CAD build for the part. Positions are in the model's coordinates, mm. A direction names the side the tool comes from. Give positions to 0.01 mm unless a question says otherwise; leave off trailing zeros. Write each loop counter-clockwise with the first axis right and the second up, starting at its lowest first coordinate (ties: lowest second). Pieces come first, ordered by that corner, then holes. Notation, with made-up numbers: (-27.75, -33.75) -> (-8.75, -33.75) arc R13 ccw to (-8.75, -25.75) -> close; hole circle Ø8 at (-34.5, 12). An arc over 180 degrees is marked (long way). Answer as a JSON object with one key per item and string values.
```python
from build123d import *

# Parameters (mm, degrees)
BOSS_EXTRUDE1_DEPTH      = 50
BOSS_EXTRUDE1_DEPTH_BACK = 50
SKETCH2_R                = 100
CUT_EXTRUDE1_DEPTH       = 50
CUT_EXTRUDE1_DEPTH_BACK  = 50
SKETCH3_R                = 75
CUT_EXTRUDE2_DEPTH       = 40
CUT_EXTRUDE2_DEPTH_BACK  = 40
SKETCH4_R                = 200


with BuildPart() as part:
    # Sketch2 → Boss-Extrude1 (new, two sides: drawn at the far end of the back side and taken through both)
    with BuildSketch(Plane.XY.offset(-BOSS_EXTRUDE1_DEPTH_BACK)):
        Circle(SKETCH2_R)
        with BuildLine():
            Line((600, 100), (0, 100))
            ThreePointArc((0, 100), (70.710678119, 70.710678119), (100, 0))
            ThreePointArc((100, 0), (70.710678119, -70.710678119), (0, -100))
            Line((0, -100), (600, -100))
            ThreePointArc((600, -100), (500, 0), (600, 100))
        make_face()
        with Locations((600, 0)):
            Circle(SKETCH2_R)
    extrude(amount=BOSS_EXTRUDE1_DEPTH + BOSS_EXTRUDE1_DEPTH_BACK)

    # Sketch3 → Cut-Extrude1 (cut, two sides: drawn at the far end of the back side and taken through both)
    with BuildSketch(Plane.XY.offset(-CUT_EXTRUDE1_DEPTH_BACK)):
        Circle(SKETCH3_R)
    extrude(amount=CUT_EXTRUDE1_DEPTH + CUT_EXTRUDE1_DEPTH_BACK, mode=Mode.SUBTRACT)

    # Sketch4 → Cut-Extrude2 (cut, two sides: drawn at the far end of the back side and taken through both)
    with BuildSketch(Plane.XY.offset(-CUT_EXTRUDE2_DEPTH_BACK)):
        Circle(SKETCH4_R)
    extrude(amount=CUT_EXTRUDE2_DEPTH + CUT_EXTRUDE2_DEPTH_BACK, mode=Mode.SUBTRACT)


solid = part.part
```
1) Slice it at A-A (y = 0). List the corners of the cut face in (x, z), then the cut area to 3 significant figures.
Model answer:
{"outline": "(-100, -50) -> (-75, -50) -> (-75, -40) -> (-100, -40) -> close; (-100, 40) -> (-75, 40) -> (-75, 50) -> (-100, 50) -> close; (75, -50) -> (700, -50) -> (700, 50) -> (75, 50) -> (75, 40) -> (200, 40) -> (200, -40) -> (75, -40) -> close", "area": "53,000 mm2"}
2) Pin check, flat tips, straight feed: pin 1 (1.5 mm diameter, centred on y = 77.5, z = 8.5, fed in from -X); pin 2 (5 mm diameter, centred on y = 9.5, z = -22.5, fed in from +X); pin 3 (1.5 mm diameter, centred on y = 42.5, z = -19, fed in from +X). Stop position of each tip, or through.
Model answer:
{"pin 1": "stops at x = 184.06", "pin 2": "stops at x = 699.75", "pin 3": "stops at x = 690.87"}
3) Mould opens along Z. For faces 3 (the flat face through (383, 1, 50)), 4 (the cylindrical face through (699.976, -2.199, -0.7)), 5 (the flat face through (81, 1, -40)) say: released by +Z, released by -Z, zero draft, split by the parting line, or undercut.
Model answer:
{"face 3": "released by +Z", "face 4": "zero draft", "face 5": "undercut"}
4) Slice it at B-B (y = 54.5). List the corners of the cut face in (x, z), then the cut area to 3 significant figures.
Model answer:
{"outline": "(-83.84, -50) -> (-51.52, -50) -> (-51.52, -40) -> (-83.84, -40) -> close; (-83.84, 40) -> (-51.52, 40) -> (-51.52, 50) -> (-83.84, 50) -> close; (51.52, -50) -> (683.84, -50) -> (683.84, 50) -> (51.52, 50) -> (51.52, 40) -> (192.43, 40) -> (192.43, -40) -> (51.52, -40) -> close", "area": "52,600 mm2"}
5) Wall check: probe 1 along X at (y, z) = (0, -42.5); probe 2 along Z at (x, y) = (106, 51); probe 3 along Y at (x, z) = (-64, 41.5). Give the ranges that are in metal, low to high.
Model answer:
{"probe 1": "x = -100 to -75, 75 to 700", "probe 2": "z = -50 to -40, 40 to 50", "probe 3": "y = -76.84 to -39.1, 39.1 to 76.84"}
6) Slice it at C-C (y = 86). List the corners of the cut face in (x, z).
Model answer:
{"outline": "(-51.03, -50) -> (651.03, -50) -> (651.03, 50) -> (-51.03, 50) -> (-51.03, 40) -> (180.57, 40) -> (180.57, -40) -> (-51.03, -40) -> close"}
7) 3-axis set-ups, long thin cutter, end or side, ignore diameter. For faces 1 (the flat face through (362, -100, -1)), 2 (the cylindrical face through (199.995, -1.466, -0.56)): which of +Z, -Z, +X, -X, +Y, -Y reach the whole face in a straight line?
Model answer:
{"face 1": "+Z, -Z, +X, -X, -Y", "face 2": "-X"}
8) Slice it at D-D (z = 17.5). List the corners of the cut face in (x, y).
Model answer:
{"outline": "(173.21, -100) -> (600, -100) arc R100 ccw to (600, 100) -> (173.21, 100) arc R200 cw to start"}
